```python
from build123d import *

# Parameters (mm, degrees)
SKETCH3_W           = 20
SKETCH3_H           = 70
BOSS_EXTRUDE3_DEPTH = 5
CUT_EXTRUDE2_DEPTH  = 2
SKETCH6_R           = 3.57
CUT_EXTRUDE3_DEPTH  = 3
SKETCH7_R           = 1.175
SKETCH7_W           = 12.35
SKETCH7_H           = 23
CUT_EXTRUDE4_DEPTH  = 5
SKETCH8_W           = 1.25
SKETCH8_H           = 25
CUT_EXTRUDE5_DEPTH  = 30
SKETCH10_W          = 20
SKETCH10_H          = 17.885322835
CUT_EXTRUDE6_DEPTH  = 10


with BuildPart() as part:
    # Sketch3 → Boss-Extrude3 (new body)
    with BuildSketch(Plane.XY):
        Rectangle(SKETCH3_W, SKETCH3_H)
    extrude(amount=BOSS_EXTRUDE3_DEPTH)

    # Sketch4 → Cut-Extrude2 (cut)
    with BuildSketch(Plane.XY.offset(5)):
        with BuildLine():
            Line((-2.85, 24.850023256), (-1.875, 12.739206809))
            Line((-1.875, 12.739206809), (1.875, 12.739206809))
            Line((1.875, 12.739206809), (2.85, 24.850023256))
            ThreePointArc((2.85, 24.850023256), (0, 23.43), (-2.85, 24.850023256))
        make_face()
        with BuildLine():
            Line((1.875, 12.739206809), (-1.875, 12.739206809))
            ThreePointArc((-1.875, 12.739206809), (0, 10.864206809), (1.875, 12.739206809))
        make_face()
        with BuildLine():
            ThreePointArc((3.57, 27), (-1.133666618, 30.385217866), (-2.85, 24.850023256))
            Line((-2.85, 24.850023256), (2.85, 24.850023256))
            ThreePointArc((2.85, 24.850023256), (3.385217866, 25.866333382), (3.57, 27))
        make_face()
        with BuildLine():
            Line((2.85, 24.850023256), (-2.85, 24.850023256))
            ThreePointArc((-2.85, 24.850023256), (0, 23.43), (2.85, 24.850023256))
        make_face()
    extrude(amount=-CUT_EXTRUDE2_DEPTH, mode=Mode.SUBTRACT)

    # Sketch6 → Cut-Extrude3 (cut)
    with BuildSketch(Plane.XY.offset(3)):
        with Locations((0, 27)):
            Circle(SKETCH6_R)
    extrude(amount=-CUT_EXTRUDE3_DEPTH, mode=Mode.SUBTRACT)

    # Sketch7 → Cut-Extrude4 (cut)
    with BuildSketch(Plane.XY.offset(5)):
        with Locations((0, -4.18)):
            Circle(SKETCH7_R)
        with Locations((0, -31.82)):
            Circle(SKETCH7_R)
        with Locations((0, -18)):
            Rectangle(SKETCH7_W, SKETCH7_H)
    extrude(amount=-CUT_EXTRUDE4_DEPTH, mode=Mode.SUBTRACT)

    # Sketch8 → Cut-Extrude5 (cut)
    with BuildSketch(Plane(origin=(10, 0, 0), x_dir=(0, 0, -1), z_dir=(1, 0, 0))):
        with Locations((-0.625, 22.5)):
            Rectangle(SKETCH8_W, SKETCH8_H)
    extrude(amount=-CUT_EXTRUDE5_DEPTH, mode=Mode.SUBTRACT)

    # Sketch10 → Cut-Extrude6 (cut)
    with BuildSketch(Plane.XY.offset(5)):
        with Locations((0, -26.057338583)):
            Rectangle(SKETCH10_W, SKETCH10_H)
    extrude(amount=-CUT_EXTRUDE6_DEPTH, mode=Mode.SUBTRACT)


solid = part.part
```
Source: CAD feature listing. Evaluate the final solid. Frame: model axes, mm. A direction names the side the tool comes from. Give positions to 0.01 mm unless a question says otherwise; leave off trailing zeros. Loops run counter-clockwise (first coordinate to the right, second up) from the corner with the lowest first, then second, coordinate; pieces in that order, holes last. Notation, with made-up numbers: (13.25, 62) -> (20.25, 62) arc R32 cw to (20.25, 89) -> close; hole circle Ø1 at (49, 50.5). An arc over 180 degrees is marked (long way). Put each result on its own line as item: value. Start each with the question number.
1) Contact query for flat-ended pins moving along their axis: P1, Ø9.5, axis at x = 0, y = 27, coming from the +Z side; P2, Ø6, axis at x = 3, y = 27.5, coming from the -Z side; P3, Ø2.5, axis at x = -0.5, z = 3.5, coming from the -Y side. Output: stop coordinate, or through.
2) Material intervals for probe 1 along Y at (x, z) = (0, 4.35) (3 decimals); probe 2 along Y at (x, z) = (0, 2) (3 decimals); probe 3 along X at (y, z) = (27, 2.55), sorted ascending.
3) Cut plane D-D (z = 0.75). Return loops of the section in (x, y) (3 decimals).
4) Cut plane C-C (x = 0). Return loops of the section in (y, z) (3 decimals).
5) Cut plane B-B (y = -12). Return loops of the section in (x, z) (3 decimals).
6) Cut plane A-A (z = 4.3). Return loops of the section in (x, y) (3 decimals), then the cut area to 3 significant figures.
7) Reachability of faces 4 (the face through (0, 0, 0)), 5 (the face through (-6.175, -12, 3)), 6 (the face through (0, 9, 5)), 7 (the face through (2.356, 18.71, 4.014)), 8 (the face through (0, 10, 1)) from +Z, -Z, +X, -X, +Y, -Y: full face, straight path, thin tool, end or side. Return the list, or none.
8) Draft query along Y for faces 1 (the face through (10, 9, 2)), 2 (the face through (0, 18, 3)), 3 (the face through (0, 35, 3)). Return one class per face: released by +Y, released by -Y, zero draft, split by the parting line, or undercut.
Results are:
1. P1: stops at z = 5
1. P2: stops at z = 1.25
1. P3: stops at y = -6.5
2. probe 1: y = -6.5 to -5.355, -3.005 to 10.864, 30.57 to 35
2. probe 2: y = -6.5 to -5.355, -3.005 to 23.43, 30.57 to 35
2. probe 3: x = -10 to -3.57, 3.57 to 10
3. outline: (-10, -17.115) -> (-6.175, -17.115) -> (-6.175, -6.5) -> (6.175, -6.5) -> (6.175, -17.115) -> (10, -17.115) -> (10, 10) -> (-10, 10) -> close; hole circle Ø2.35 at (0, -4.18)
4. outline: (-6.5, 0) -> (-5.355, 0) -> (-5.355, 5) -> (-6.5, 5) -> close; (-3.005, 0) -> (10, 0) -> (10, 1.25) -> (23.43, 1.25) -> (23.43, 3) -> (10.864, 3) -> (10.864, 5) -> (-3.005, 5) -> close; (30.57, 1.25) -> (35, 1.25) -> (35, 5) -> (30.57, 5) -> close
5. outline: (-10, 0) -> (-6.175, 0) -> (-6.175, 5) -> (-10, 5) -> close; (6.175, 0) -> (10, 0) -> (10, 5) -> (6.175, 5) -> close
6. outline: (-10, -17.115) -> (-6.175, -17.115) -> (-6.175, -6.5) -> (6.175, -6.5) -> (6.175, -17.115) -> (10, -17.115) -> (10, 35) -> (-10, 35) -> close; hole (-2.85, 24.85) -> (-1.875, 12.739) arc R1.875 ccw to (1.875, 12.739) -> (2.85, 24.85) arc R3.57 ccw (long way) to start; hole circle Ø2.35 at (0, -4.18)
6. area: 810 mm2
7. face 4: -Z, +X, -X, +Y, -Y
7. face 5: +Z, -Z, -Y
7. face 6: +Z, +X, -X, +Y, -Y
7. face 7: +Z
7. face 8: -Z, +X, -X, +Y
8. face 1: zero draft
8. face 2: undercut
8. face 3: released by +Y
